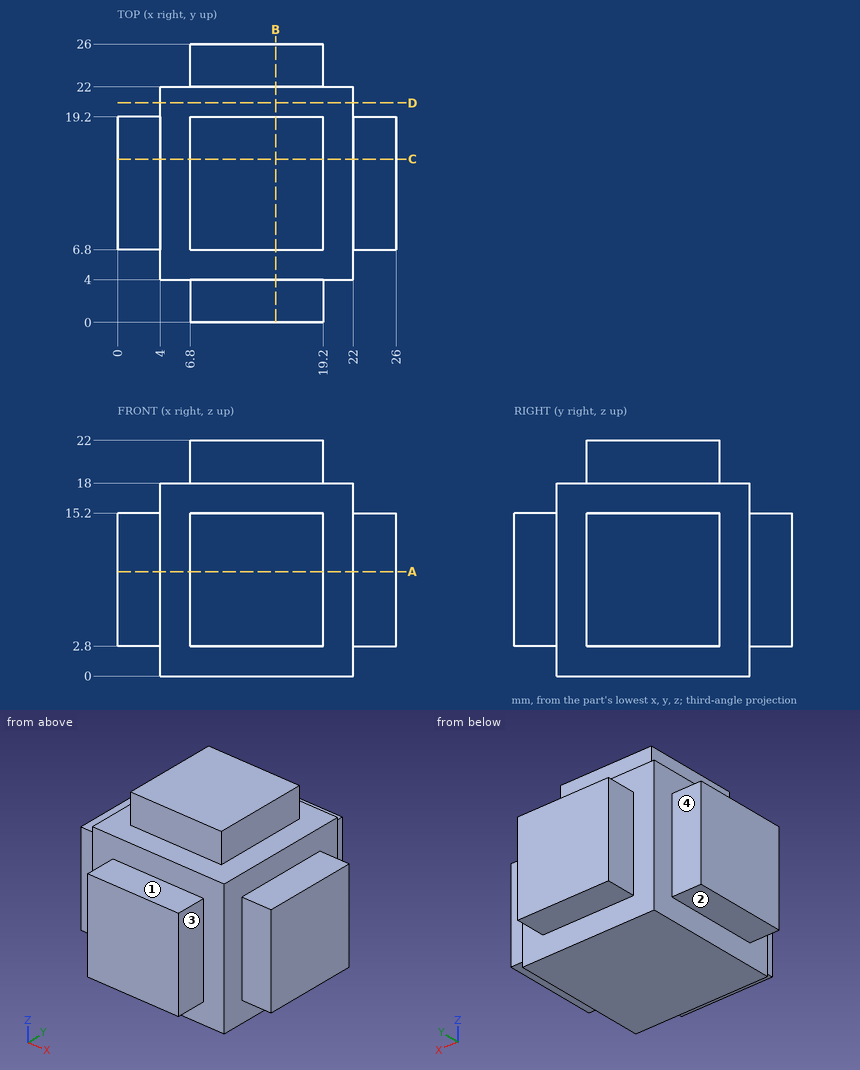
Design review of the part shown in the three views and the two pictorial views. Dimensions are in mm from the part's minimum x, y and z. A direction names the side the tool comes from. Coordinates: 2 decimals unless noted, no trailing zeros. Write each loop counter-clockwise with the first axis right and the second up, starting at its lowest first coordinate (ties: lowest second). Pieces come first, ordered by that corner, then holes.
1) We need section A-A on z = 9.75. State the section outline as (x, y) points, then the cut area to 3 significant figures.
2) Machinability: for the marked faces 1, 2, 3 and 4, which of the approach directions +Z, -Z, +X, -X, +Y, -Y give a long, thin tool a straight path to every point of the face, cutting with its end or side? Answer none if there is none.
3) We need section B-B on x = 14.75. State the section outline as (y, z) points.
4) Clearance check with flat-ended pins moving along their axes: pin 1 Ø8 at (y, z) = (22.5, 19.5) entering from -X; pin 2 Ø2 at (y, z) = (13, 20.5) entering from -X; pin 3 Ø10 at (x, y) = (23, 9) entering from -Z; pin 4 Ø1.2 at (y, z) = (11.5, 20.5) entering from +X. State where each tip first meets the part, or that it passes through.
5) To check wall thickness, follow probe 1 along Y at (x, z) = (7.5, 2.75); probe 2 along Z at (x, y) = (3.25, 14). State the ranges of each line that lie inside material, in increasing order.
6) We need section D-D on y = 20.5. State the section outline as (x, z) points.
Answer list:
1. outline: (0, 6.8) - (4, 6.8) - (4, 4) - (6.8, 4) - (6.8, 0) - (19.2, 0) - (19.2, 4) - (22, 4) - (22, 6.8) - (26, 6.8) - (26, 19.2) - (22, 19.2) - (22, 22) - (19.2, 22) - (19.2, 26) - (6.8, 26) - (6.8, 22) - (4, 22) - (4, 19.2) - (0, 19.2) - close
1. area: 522 mm2
2. face 1: +Z, +X, -X, -Y
2. face 2: -Z, -X, +Y, -Y
2. face 3: +Z, -Z, +X, -Y
2. face 4: +Z, -Z, -X, +Y
3. outline: (0, 2.8) - (4, 2.8) - (4, 0) - (22, 0) - (22, 2.8) - (26, 2.8) - (26, 15.2) - (22, 15.2) - (22, 18) - (19.2, 18) - (19.2, 22) - (6.8, 22) - (6.8, 18) - (4, 18) - (4, 15.2) - (0, 15.2) - close
4. pin 1: stops at x = 4
4. pin 2: stops at x = 6.8
4. pin 3: stops at z = 0
4. pin 4: stops at x = 19.2
5. probe 1: y = 4 to 22
5. probe 2: z = 2.8 to 15.2
6. outline: (4, 0) - (22, 0) - (22, 18) - (4, 18) - close
